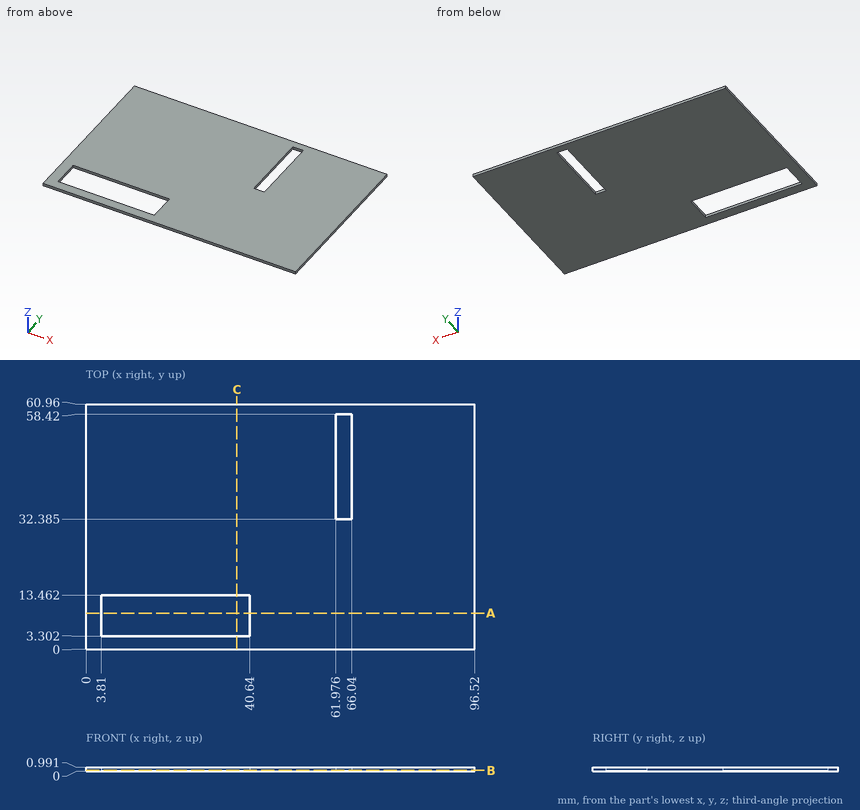
Could you check a few things on this drawing? It's one solid part, dimensions in mm from its lowest x, y, z. Coordinates: 2 decimals unless noted, no trailing zeros. Order: outer loops, then holes, each group sorted by start corner. A loop starts at its lowest first (then second) coordinate and runs counter-clockwise, first axis right, second up. Notation, with made-up numbers: M 68,-13 L 76,-13 A22 ccw 76,-1 Z; hole C 24,-17.5 d1. An arc over 180 degrees is marked long. Use a Markdown table: item, result. Add a question column.
Q1. If I drill on L1, parallel to X at y = 46.5, z = 0.55; L2, parallel to Y at x = 37.5, z = 0.1; L3, parallel to Y at x = 66, z = 0.75 (1 decimal), over which ranges is the centre line in solid material (lowest first)?
Q2. I want a section at A-A on y = 9. List the corners of the cut face in (x, z) for me.
Q3. I'm going to push a flat-ended pin straight in: pin 1 (0.5 mm diameter, centred on y = 10, z = 0.5, fed in from -X). Where does the tip first touch, or does it pass through?
Q4. I want a section at B-B on z = 0.25. List the corners of the cut face in (x, y) for me (1 decimal), then the cut area to 3 significant figures.
Q5. I want a section at C-C on x = 37.5. List the corners of the cut face in (y, z) for me.
Checked values:
| question | item | result |
|---|---|---|
| 1 | L1 | 0 to 61.98, 66.04 to 96.52 |
| 1 | L2 | 0 to 3.3, 13.46 to 60.96 |
| 1 | L3 | 0 to 32.4, 58.4 to 61 |
| 2 | outline | M 0,0 L 3.81,0 L 3.81,0.99 L 0,0.99 Z; M 40.64,0 L 96.52,0 L 96.52,0.99 L 40.64,0.99 Z |
| 3 | pin 1 | x = 0 |
| 4 | outline | M 0,0 L 96.5,0 L 96.5,61 L 0,61 Z; hole M 3.8,3.3 L 40.6,3.3 L 40.6,13.5 L 3.8,13.5 Z; hole M 62,32.4 L 66,32.4 L 66,58.4 L 62,58.4 Z |
| 4 | area | 5,400 mm² |
| 5 | outline | M 0,0 L 3.3,0 L 3.3,0.99 L 0,0.99 Z; M 13.46,0 L 60.96,0 L 60.96,0.99 L 13.46,0.99 Z |
